Source: CAD feature listing. Evaluate the final solid. Frame: model axes, mm. A direction names the side the tool comes from. Round coordinates to 2 decimals unless told otherwise and drop trailing zeros.
from build123d import *

# Parameters (mm, degrees)
SKETCH1_W                     = 8.5
SKETCH1_H                     = 6.35
BOSS_EXTRUDE1_DEPTH           = 1.89
BOSS_EXTRUDE1_TAPER           = 5
BOSS_EXTRUDE1_OTHER_WAY_DEPTH = 2.49
BOSS_EXTRUDE1_OTHER_WAY_TAPER = 5
SKETCH2_W                     = 1.4
SKETCH2_H                     = 0.25
LPATTERN1_COUNT               = 2
LPATTERN1_PITCH               = 2.54
LPATTERN1_COL_COUNT           = 2
LPATTERN1_COL_PITCH           = 2.54
MIRROR1_COPY_1_SKETCH_W       = 1.4
MIRROR1_COPY_1_SKETCH_H       = 0.25
MIRROR1_COPY_2_SKETCH_W       = 1.4
MIRROR1_COPY_2_SKETCH_H       = 0.25
SKETCH4_R                     = 0.606643951
CUT_EXTRUDE1_DEPTH            = 0.25


with BuildPart() as part:
    # Sketch1 → Boss-Extrude1 (new body)
    with BuildSketch(Plane(origin=(0, 0, 0), x_dir=(1, 0, 0), z_dir=(0, 1, 0))):
        Rectangle(SKETCH1_W, SKETCH1_H)
    extrude(amount=BOSS_EXTRUDE1_DEPTH, taper=BOSS_EXTRUDE1_TAPER)

    # Sketch1 → Boss-Extrude1 other way (add)
    with BuildSketch(Plane(origin=(0, 0, 0), x_dir=(1, 0, 0), z_dir=(0, 1, 0))):
        Rectangle(SKETCH1_W, SKETCH1_H)
    extrude(amount=-BOSS_EXTRUDE1_OTHER_WAY_DEPTH, taper=BOSS_EXTRUDE1_OTHER_WAY_TAPER)

    # Sweep1: sweep along a path in Sketch3
    with BuildLine(Plane(origin=(0, 0, 0), x_dir=(0, 0, -1), z_dir=(1, 0, 0))) as sweep1_path:
        Line((0, 0), (-3.3139807, 0))
        ThreePointArc((-3.3139807, 0), (-3.577719026, -0.099264077), (-3.710558645, -0.347789523))
        Line((-3.710558645, -0.347789523), (-3.996826594, -2.522210477))
        ThreePointArc((-3.996826594, -2.522210477), (-4.129666213, -2.770735923), (-4.393404539, -2.87))
        Line((-4.393404539, -2.87), (-4.75, -2.87))
    # Sketch2 → Sweep1 (sweep)
    with BuildSketch(Plane.XY):
        Rectangle(SKETCH2_W, SKETCH2_H)
    sweep1 = sweep(path=sweep1_path.line)

    # LPattern1: Sweep1 ×2
    with Locations(*[(i * LPATTERN1_PITCH, 0, 0) for i in range(1, LPATTERN1_COUNT)]):
        add(sweep1)

    # LPattern1 col: Sweep1 ×2
    with Locations(*[(-i * LPATTERN1_COL_PITCH, 0, 0) for i in range(1, LPATTERN1_COL_COUNT)]):
        add(sweep1)

    # Mirror1: Sweep1 across plane
    add(sweep1.mirror(Plane.XY))

    # Mirror1 copy 1: sweep along a path in Mirror1 copy 1 path
    with BuildLine(Plane(origin=(2.54, 0, 0), x_dir=(0, 0, 1), z_dir=(1, 0, 0))) as mirror1_copy_1_path:
        Line((0, 0), (-3.3139807, 0))
        ThreePointArc((-3.3139807, 0), (-3.577719026, 0.099264077), (-3.710558645, 0.347789523))
        Line((-3.710558645, 0.347789523), (-3.996826594, 2.522210477))
        ThreePointArc((-3.996826594, 2.522210477), (-4.129666213, 2.770735923), (-4.393404539, 2.87))
        Line((-4.393404539, 2.87), (-4.75, 2.87))
    # Mirror1 copy 1 sketch → Mirror1 copy 1 (sweep)
    with BuildSketch(Plane(origin=(2.54, 0, 0), x_dir=(1, 0, 0), z_dir=(0, 0, -1))):
        Rectangle(MIRROR1_COPY_1_SKETCH_W, MIRROR1_COPY_1_SKETCH_H)
    sweep(path=mirror1_copy_1_path.line)

    # Mirror1 copy 2: sweep along a path in Mirror1 copy 2 path
    with BuildLine(Plane(origin=(-2.54, 0, 0), x_dir=(0, 0, 1), z_dir=(1, 0, 0))) as mirror1_copy_2_path:
        Line((0, 0), (-3.3139807, 0))
        ThreePointArc((-3.3139807, 0), (-3.577719026, 0.099264077), (-3.710558645, 0.347789523))
        Line((-3.710558645, 0.347789523), (-3.996826594, 2.522210477))
        ThreePointArc((-3.996826594, 2.522210477), (-4.129666213, 2.770735923), (-4.393404539, 2.87))
        Line((-4.393404539, 2.87), (-4.75, 2.87))
    # Mirror1 copy 2 sketch → Mirror1 copy 2 (sweep)
    with BuildSketch(Plane(origin=(-2.54, 0, 0), x_dir=(1, 0, 0), z_dir=(0, 0, -1))):
        Rectangle(MIRROR1_COPY_2_SKETCH_W, MIRROR1_COPY_2_SKETCH_H)
    sweep(path=mirror1_copy_2_path.line)

    # Sketch4 → Cut-Extrude1 (cut)
    with BuildSketch(Plane(origin=(0, 1.89, 0), x_dir=(1, 0, 0), z_dir=(0, 1, 0))):
        with Locations(Location((-2.903482354, -1.641715186, 0), (0, 0, 270))):
            Circle(SKETCH4_R)
    extrude(amount=-CUT_EXTRUDE1_DEPTH, mode=Mode.SUBTRACT)


solid = part.part
1) Contact query for flat-ended pins moving along their axis: P1, Ø0.8, axis at y = -2, z = -4, coming from the -X side; P2, Ø1.6, axis at x = -2.9, z = 1.64, coming from the -Y side; P3, Ø0.6, axis at x = -2.5, z = 1.5, coming from the +Y side; P4, Ø1.7, axis at y = -1, z = 4, coming from the +X side. Output: stop coordinate, or through.
Taken from the geometry:
P1: stops at x = -3.24
P2: stops at y = -2.49
P3: stops at y = 1.89
P4: stops at x = 3.24
2) Section query A-A on y = -2. State how many separate pieces and enclosed holes the cut face has, then the cut area to 3 significant figures.
Taken from the geometry:
separate pieces: 7
enclosed holes: 0
area: 51.0 mm2
3) Reachability of faces 1 (the face through (-0.01, -1.467, 3.732)), 2 (the face through (-2.53, -1.43, 3.98)) from +Z, -Z, +X, -X, +Y, -Y: full face, straight path, thin tool, end or side. Return the list, or none.
Taken from the geometry:
face 1: +X, -X, -Y
face 2: +Z, +X, -X, +Y
4) Material intervals for line 1 (X direction, y = -1.85, z = -4); line 2 (Z direction, x = -2.5, y = -0.65); line 3 (Z direction, x = 0.5, y = -2.4), sorted ascending.
Taken from the geometry:
line 1: x = -3.24 to -1.84, -0.7 to 0.7, 1.84 to 3.24
line 2: z = -3.88 to -3.62, -3.12 to 3.12, 3.62 to 3.88
line 3: z = -4.11 to -3.85, -2.97 to 2.97, 3.85 to 4.11
